from build123d import *

# Parameters (mm, degrees)
BOSS_EXTRUDE1_DEPTH     = 5
CUT_EXTRUDE1_DEPTH      = 12.517223111
CUT_EXTRUDE1_DEPTH_BACK = 12.517223111
SKETCH2_W               = 2.2
SKETCH2_H               = 5.949489743
BOSS_EXTRUDE2_DEPTH     = 5


with BuildPart() as part:
    # Sketch1 → Boss-Extrude1 (new body)
    with BuildSketch(Plane.XY):
        with BuildLine():
            Line((-7.5, 5.949489743), (2.5, 5.949489743))
            Line((2.5, 5.949489743), (2.5, 2.449489743))
            ThreePointArc((2.5, 2.449489743), (3.226702194, -1.355873501), (0, -3.5))
            Line((0, -3.5), (-5, -3.5))
            ThreePointArc((-5, -3.5), (-8.226702194, -1.355873501), (-7.5, 2.449489743))
            Line((-7.5, 2.449489743), (-7.5, 5.949489743))
        make_face()
    extrude(amount=BOSS_EXTRUDE1_DEPTH)

    # Sketch2 → Cut-Extrude1 (cut, two sides: drawn at the far end of the back side and taken through both)
    with BuildSketch(Plane(origin=(0, 0, 0), x_dir=(0, 0, -1), z_dir=(1, 0, 0)).offset(-CUT_EXTRUDE1_DEPTH_BACK)):
        with Locations((-2.5, -0.525255129)):
            Rectangle(SKETCH2_W, SKETCH2_H)
    extrude(amount=CUT_EXTRUDE1_DEPTH + CUT_EXTRUDE1_DEPTH_BACK, mode=Mode.SUBTRACT)

    # Sketch3 → Boss-Extrude2 (add)
    with BuildSketch(Plane.XY):
        with BuildLine():
            Line((-5, -2.179025152), (0, -2.179025152))
            ThreePointArc((0, -2.179025152), (1.5, -0.679025152), (0, 0.820974848))
            Line((0, 0.820974848), (-5, 0.820974848))
            ThreePointArc((-5, 0.820974848), (-6.5, -0.679025152), (-5, -2.179025152))
        make_face()
    extrude(amount=BOSS_EXTRUDE2_DEPTH)


solid = part.part
Design review of the part built by this model. Coordinates are the model's own, in mm. A direction names the side the tool comes from. Round coordinates to 2 decimals unless told otherwise and drop trailing zeros. Write each loop counter-clockwise with the first axis right and the second up, starting at its lowest first coordinate (ties: lowest second). Pieces come first, ordered by that corner, then holes. Notation, with made-up numbers: (88, 38.5) - (114, 38.5) arc R17 ccw to (114, 63.5) - close; hole circle Ø8 at (-18, 51.25). An arc over 180 degrees is marked (long way). Use a Markdown table: item, result. Add a question column.
1. We need section B-B (y = 1.5). State the section outline as (x, z) points.
2. Wall thickness on probe 1 along Y at (x, z) = (-1.25, 2.3); probe 2 along Z at (x, y) = (1.75, -1); probe 3 along X at (y, z) = (-0.75, 1.5): over which ranges is each line inside the solid? List them lowest first.
3. We need section D-D (z = 3.8). State the section outline as (x, y) points.
4. Mouldability with a two-part tool opening along Z and no side actions: class faces 5 (the face through (-3, 2.449, 3)), 6 (the face through (-3, 1, 0)), 7 (the face through (-2, 1, 5)), 8 (the face through (-7.5, 4, 2)) as +Z half, -Z half, draft (parallel to the pull), parting line (faces both ways), or undercut.
5. For faces 1 (the face through (1.5, -0.7, 2.5)), 2 (the face through (-6.5, -0.65, 2.48)), 3 (the face through (-3, -2.179, 2)), 4 (the face through (-3, 1, 1.4)), list the 3-axis set-ups (+Z, -Z, +X, -X, +Y, -Y) from which the entire face can be reached by the end or side of a thin tool; tool diameter is ignored.
6. We need section A-A (z = 2.35). State the section outline as (x, y) points.
7. Clearance check with flat-ended pins moving along their axes: pin 1 (1.5 mm diameter, centred on y = 1, z = 2.5, fed in from -X); pin 2 (1.8 mm diameter, centred on x = -2.5, z = 2.5, fed in from -Y); pin 3 (1 mm diameter, centred on y = 5, z = 2, fed in from +X). State where each tip first meets the part, or that it passes through.
8. We need section C-C (x = -3.25). State the section outline as (y, z) points, then the cut area to 3 significant figures.
Output:
| question | item | result |
|---|---|---|
| 1 | outline | (-8.16, 0) - (3.16, 0) - (3.16, 1.4) - (-8.16, 1.4) - close; (-8.16, 3.6) - (3.16, 3.6) - (3.16, 5) - (-8.16, 5) - close |
| 2 | probe 1 | y = -2.18 to 0.82, 2.45 to 5.95 |
| 2 | probe 2 | z = 0 to 1.4, 3.6 to 5 |
| 2 | probe 3 | x = -6.5 to 1.5 |
| 3 | outline | (-7.5, 2.45) arc R3.5 ccw to (-5, -3.5) - (0, -3.5) arc R3.5 ccw to (2.5, 2.45) - (2.5, 5.95) - (-7.5, 5.95) - close |
| 4 | face 5 | undercut |
| 4 | face 6 | -Z half |
| 4 | face 7 | +Z half |
| 4 | face 8 | draft |
| 5 | face 1 | +X |
| 5 | face 2 | -X |
| 5 | face 3 | +X, -X, -Y |
| 5 | face 4 | none |
| 6 | outline | (-7.5, 2.45) - (2.5, 2.45) - (2.5, 5.95) - (-7.5, 5.95) - close; (-5, -2.18) - (0, -2.18) arc R1.5 ccw to (0, 0.82) - (-5, 0.82) arc R1.5 ccw to start |
| 7 | pin 1 | stops at x = -6.18 |
| 7 | pin 2 | stops at y = -2.18 |
| 7 | pin 3 | stops at x = 2.5 |
| 8 | outline | (-3.5, 0) - (5.95, 0) - (5.95, 5) - (-3.5, 5) - (-3.5, 3.6) - (-2.18, 3.6) - (-2.18, 1.4) - (-3.5, 1.4) - close; hole (0.82, 1.4) - (2.45, 1.4) - (2.45, 3.6) - (0.82, 3.6) - close |
| 8 | area | 40.8 mm2 |
